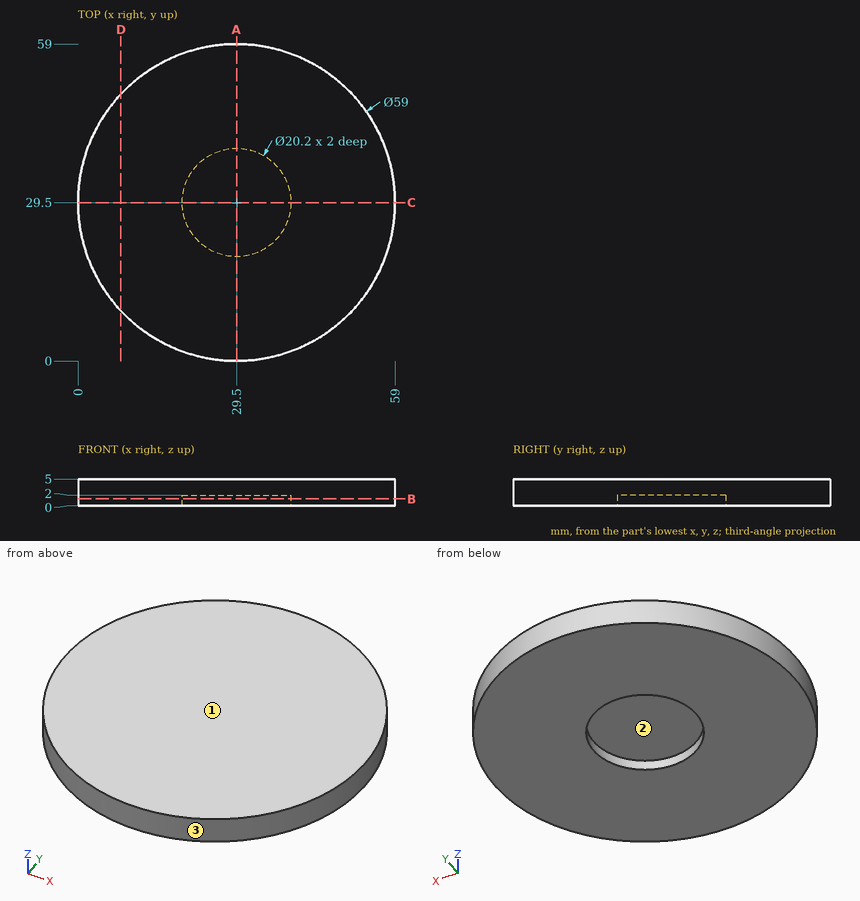
Geometry check sheet. Reference: drawing and pictorial views, mm from the part's lowest x, y, z. Round coordinates to 2 decimals unless told otherwise and drop trailing zeros. Loops run counter-clockwise (first coordinate to the right, second up) from the corner with the lowest first, then second, coordinate; pieces in that order, holes last. Notation, with made-up numbers: M 31,-26.5 L 36,-26.5 A33 cw 36,5.5 Z; hole C 89.5,30 d8. An arc over 180 degrees is marked long. Return JSON: item names as keys, results as strings. Group by question number.
(1) Section check B-B, the plane z = 1.3. Enter the section's corners in (x, y), and give its area (3 significant figures).
(2) Section check A-A, the plane x = 29.5. Enter the section's corners in (y, z).
(3) Section check D-D, the plane x = 8. Enter the section's corners in (y, z), and give its area (3 significant figures).
(4) Scan lines: line 1 along Y through (x, z) = (29.5, 1.25); line 2 along Y through (x, z) = (29.5, 3.3); line 3 along Z through (x, y) = (37.5, 24). Record each from-to range of solid material in increasing order. Write a range as [from, to].
(5) Go/stop test with flat-tipped pins: pin 1 (6 mm diameter, centred on x = 26, y = 29.5, fed in from -Z); pin 2 (1.5 mm diameter, centred on x = 40.5, z = 2, fed in from -Y); pin 3 (3 mm diameter, centred on y = 19.5, z = 2, fed in from +X). Record where each tip stops, or that it passes through.
(6) Mould release check, pull along X, two halves, no side actions. Record for the marked faces 1, 2 and 3: pulls with the +X half, pulls with the -X half, needs draft (parallel to the pull), parting line crosses it, or undercut.
Data:
{
 "1": {"outline": "C 29.5,29.5 d59; hole C 29.5,29.5 d20.2", "area": "2,410 mm²"},
 "2": {"outline": "M 0,0 L 19.4,0 L 19.4,2 L 39.6,2 L 39.6,0 L 59,0 L 59,5 L 0,5 Z"},
 "3": {"outline": "M 9.3,0 L 49.7,0 L 49.7,5 L 9.3,5 Z", "area": "202 mm²"},
 "4": {"line 1": "[0, 19.4], [39.6, 59]", "line 2": "[0, 59]", "line 3": "[2, 5]"},
 "5": {"pin 1": "z = 2", "pin 2": "y = 1.84", "pin 3": "x = 57.75"},
 "6": {"face 1": "needs draft", "face 2": "undercut", "face 3": "parting line crosses it"}
}
